Design review of the part built by this model. Coordinates are the model's own, in mm. Face numbers are marked on the shaded views. A direction names the side the tool comes from. Give positions to 0.01 mm unless a question says otherwise; leave off trailing zeros. Loops run counter-clockwise (first coordinate to the right, second up) from the corner with the lowest first, then second, coordinate; pieces in that order, holes last. Notation, with made-up numbers: (87.25, 65.5) -> (132.25, 65.5) arc R31 ccw to (132.25, 96.5) -> close; hole circle Ø4 at (11, 88.25). An arc over 180 degrees is marked (long way). Answer in a Markdown table with one row per item. Add a question column.
(1) Consider section B-B on y = -38.1. Write out the cut boundary in (x, z).
(2) Consider section D-D on y = -72. Write out the cut boundary in (x, z).
(3) Consider section C-C on z = 8. Write out the cut boundary in (x, y), then the cut area to 3 significant figures.
(4) Draft analysis for pull direction Z (two halves, no side actions). For the marked faces 1, 2 and 3, state which applies: +Z half, -Z half, draft (parallel to the pull), parting line (faces both ways), or undercut.
(5) For pin 1 (4 mm diameter, centred on x = -25.5, y = -83, fed in from +Z); pin 2 (12 mm diameter, centred on y = -42.5, z = 0.5, fed in from +X); pin 3 (14 mm diameter, centred on x = -20, y = -80.5, fed in from -Z); pin 4 (6 mm diameter, centred on x = 15, z = 8, fed in from -Y), all flat-tipped, find the tip position at first contact; note any pin that passes through.
(6) Consider section A-A on x = -19. Write out the cut boundary in (y, z), then the cut area to 3 significant figures.
(7) For line 1 (Y direction, x = -48, z = 38); line 2 (X direction, y = -19.5, z = 36); line 3 (Z direction, x = 20, y = -47), list the stretches that pass through material, from the lowest coordinate up.
(8) For the marked faces 4, 5 and 6, list the 3-axis set-ups (+Z, -Z, +X, -X, +Y, -Y) from which the entire face can be reached by the end or side of a thin tool; tool diameter is ignored.
from build123d import *

# Parameters (mm, degrees)
F0_W     = 76.2
F0_H     = 76.2
F1_DEPTH = 76.2
F2_W     = 25.4
F2_H     = 25.4
F3_DEPTH = 12.7
F4_R     = 12.7
F5_DEPTH = 25.4
F6_DEPTH = 25.4


with BuildPart() as f1:
    # F0 (on Front) → F1 (new body)
    with BuildSketch(Plane.XZ):
        with Locations((-25.176713, 26.619935)):
            Rectangle(F0_W, F0_H)
    extrude(amount=F1_DEPTH)

    # F2 (on face) → F3 (join)
    with BuildSketch(Plane.XZ.offset(76.2)):
        with Locations((-25.176713, 26.619935)):
            Rectangle(F2_W, F2_H)
    extrude(amount=F3_DEPTH)

    # F4 (on face) → F5 (join)
    with BuildSketch(Plane.YZ.offset(12.923287)):
        with Locations((-38.1, 37.798271)):
            Circle(F4_R)
    extrude(amount=F5_DEPTH)

    # F4 (on face) → F6 (join)
    with BuildSketch(Plane.YZ.offset(12.923287)):
        with Locations((-38.1, 37.798271)):
            Circle(F4_R)
    extrude(amount=F6_DEPTH)


solid = f1.part
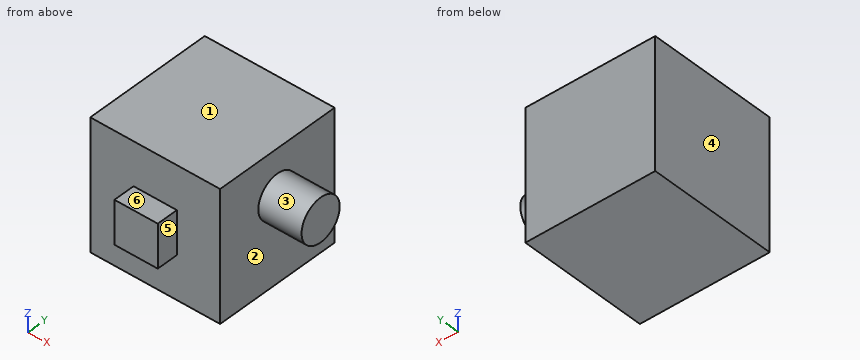
Values follow:
| question | item | result |
|---|---|---|
| 1 | outline | (-63.28, -11.48) -> (12.92, -11.48) -> (12.92, 25.1) -> (38.32, 25.1) -> (38.32, 50.5) -> (12.92, 50.5) -> (12.92, 64.72) -> (-63.28, 64.72) -> close |
| 2 | outline | (-63.28, -11.48) -> (12.92, -11.48) -> (12.92, 64.72) -> (-63.28, 64.72) -> close |
| 3 | outline | (-63.28, -76.2) -> (12.92, -76.2) -> (12.92, 0) -> (-63.28, 0) -> close |
| 3 | area | 5,810 mm2 |
| 4 | face 1 | +Z half |
| 4 | face 2 | draft |
| 4 | face 3 | parting line |
| 5 | pin 1 | z = 39.32 |
| 5 | pin 2 | x = 12.92 |
| 5 | pin 3 | z = -11.48 |
| 5 | pin 4 | y = -76.2 |
| 6 | outline | (-88.9, 13.92) -> (-76.2, 13.92) -> (-76.2, -11.48) -> (0, -11.48) -> (0, 64.72) -> (-76.2, 64.72) -> (-76.2, 39.32) -> (-88.9, 39.32) -> close |
| 6 | area | 6,130 mm2 |
| 7 | line 1 | -76.2 to 0 |
| 7 | line 2 | -63.28 to 12.92 |
| 7 | line 3 | 28.74 to 46.86 |
| 8 | face 4 | +Z, -Z, -X, +Y, -Y |
| 8 | face 5 | +Z, -Z, +X, -Y |
| 8 | face 6 | +Z, +X, -X, -Y |
